Autodesk Inventor part; units mm, degrees
ref_plane "YZ Plane" through (0, 0, 0) normal (1, 0, 0) x (0, 1, 0)
ref_plane "XZ Plane" through (0, 0, 0) normal (0, 1, 0) x (-1, 0, 0)
ref_plane "XY Plane" through (0, 0, 0) normal (0, 0, 1) x (1, 0, 0)
sketch "Sketch1" plane through (0, 0, 0) normal (0, 0, 1) x (1, 0, 0)
  line L0 (0, 0) -> (762, 0)
  line L1 (0, 0) -> (0, -101.6)
  line L2 (0, -101.6) -> (76.2, -101.6)
  line L3 (76.2, -101.6) -> (76.2, -203.2)
  line L4 (76.2, -203.2) -> (0, -203.2)
  line L5 (0, -203.2) -> (0, -266.7)
  line L6 (0, -266.7) -> (228.6, -266.7)
  line L7 (228.6, -266.7) -> (228.6, -355.6)
  line L8 (0, -711.2) -> (762, -711.2)
  line L9 (0, -711.2) -> (0, -609.6)
  line L10 (0, -609.6) -> (76.2, -609.6)
  line L11 (76.2, -609.6) -> (76.2, -508)
  line L12 (76.2, -508) -> (0, -508)
  line L13 (0, -508) -> (0, -444.5)
  line L14 (0, -444.5) -> (228.6, -444.5)
  line L15 (228.6, -444.5) -> (228.6, -355.6)
  line L16 (762, 0) -> (762, -101.6)
  line L17 (762, -101.6) -> (685.8, -101.6)
  line L18 (685.8, -101.6) -> (685.8, -203.2)
  line L19 (685.8, -203.2) -> (762, -203.2)
  line L20 (762, -203.2) -> (762, -266.7)
  line L21 (762, -266.7) -> (533.4, -266.7)
  line L22 (533.4, -266.7) -> (533.4, -355.6)
  line L23 (762, -711.2) -> (762, -609.6)
  line L24 (762, -609.6) -> (685.8, -609.6)
  line L25 (685.8, -609.6) -> (685.8, -508)
  line L26 (685.8, -508) -> (762, -508)
  line L27 (762, -508) -> (762, -444.5)
  line L28 (762, -444.5) -> (533.4, -444.5)
  line L29 (533.4, -444.5) -> (533.4, -355.6)
  dimension "d0" = 762
  dimension "d1" = 101.6
  dimension "d2" = 76.2
  dimension "d3" = 101.6
  dimension "d4" = 63.5
  dimension "d5" = 228.6
  dimension "d7" = 88.9
extrude "Extrusion1" add sketch "Sketch1" along normal blind 9.525
sketch "Sketch2" plane through (0, 0, 9.525) normal (0, 0, 1) x (1, 0, 0)
  line L0 (0, 0) -> (12.7, 0)
  line L1 (0, 0) -> (762, 0)
  line L2 (12.7, 0) -> (12.7, -12.7)
  line L3 (12.7, -12.7) -> (38.1, -12.7)
  line L4 (38.1, -12.7) -> (38.1, -38.1)
  line L5 (38.1, -38.1) -> (12.7, -38.1)
  circle A0 centre (12.7, -12.7) radius 2.54
  circle A1 centre (38.1, -12.7) radius 2.54
  circle A2 centre (38.1, -38.1) radius 2.54
  circle A3 centre (12.7, -38.1) radius 2.54
  line L6 (0, -203.2) -> (76.2, -203.2)
  line L7 (0, -203.2) -> (12.7, -203.2)
  line L8 (12.7, -203.2) -> (12.7, -215.9)
  line L9 (228.6, -266.7) -> (0, -266.7)
  line L10 (0, -266.7) -> (12.7, -266.7)
  line L11 (12.7, -266.7) -> (12.7, -254)
  circle A4 centre (12.7, -254) radius 2.54
  circle A5 centre (12.7, -215.9) radius 2.54
  line L12 (381, 0) -> (381, -711.2)
  line L13 (762, -711.2) -> (0, -711.2)
  line L14 (0, -355.6) -> (762, -355.6)
  line L15 (762, 0) -> (749.3, 0)
  line L16 (762, 0) -> (0, 0)
  line L17 (749.3, 0) -> (749.3, -12.7)
  line L18 (749.3, -12.7) -> (723.9, -12.7)
  line L19 (723.9, -12.7) -> (723.9, -38.1)
  line L20 (723.9, -38.1) -> (749.3, -38.1)
  circle A6 centre (749.3, -12.7) radius 2.54
  circle A7 centre (723.9, -12.7) radius 2.54
  circle A8 centre (723.9, -38.1) radius 2.54
  circle A9 centre (749.3, -38.1) radius 2.54
  line L21 (762, -203.2) -> (685.8, -203.2)
  line L22 (762, -203.2) -> (749.3, -203.2)
  line L23 (749.3, -203.2) -> (749.3, -215.9)
  line L24 (533.4, -266.7) -> (762, -266.7)
  line L25 (762, -266.7) -> (749.3, -266.7)
  line L26 (749.3, -266.7) -> (749.3, -254)
  circle A10 centre (749.3, -254) radius 2.54
  circle A11 centre (749.3, -215.9) radius 2.54
  line L27 (0, -711.2) -> (12.7, -711.2)
  line L28 (0, -711.2) -> (762, -711.2)
  line L29 (12.7, -711.2) -> (12.7, -698.5)
  line L30 (12.7, -698.5) -> (38.1, -698.5)
  line L31 (38.1, -698.5) -> (38.1, -673.1)
  line L32 (38.1, -673.1) -> (12.7, -673.1)
  circle A12 centre (12.7, -698.5) radius 2.54
  circle A13 centre (38.1, -698.5) radius 2.54
  circle A14 centre (38.1, -673.1) radius 2.54
  circle A15 centre (12.7, -673.1) radius 2.54
  line L33 (0, -508) -> (76.2, -508)
  line L34 (0, -508) -> (12.7, -508)
  line L35 (12.7, -508) -> (12.7, -495.3)
  line L36 (228.6, -444.5) -> (0, -444.5)
  line L37 (0, -444.5) -> (12.7, -444.5)
  line L38 (12.7, -444.5) -> (12.7, -457.2)
  circle A16 centre (12.7, -457.2) radius 2.54
  circle A17 centre (12.7, -495.3) radius 2.54
  line L39 (381, -711.2) -> (381, 0)
  line L40 (762, -711.2) -> (749.3, -711.2)
  line L41 (762, -711.2) -> (0, -711.2)
  line L42 (749.3, -711.2) -> (749.3, -698.5)
  line L43 (749.3, -698.5) -> (723.9, -698.5)
  line L44 (723.9, -698.5) -> (723.9, -673.1)
  line L45 (723.9, -673.1) -> (749.3, -673.1)
  circle A18 centre (749.3, -698.5) radius 2.54
  line L46 (533.4, -444.5) -> (762, -444.5)
  line L47 (749.3, -444.5) -> (749.3, -457.2)
  line L48 (762, -444.5) -> (749.3, -444.5)
  circle A19 centre (749.3, -457.2) radius 2.54
  circle A20 centre (749.3, -495.3) radius 2.54
  line L49 (749.3, -508) -> (749.3, -495.3)
  line L50 (762, -508) -> (685.8, -508)
  line L51 (762, -508) -> (749.3, -508)
  circle A21 centre (723.9, -673.1) radius 2.54
  circle A22 centre (723.9, -698.5) radius 2.54
  circle A23 centre (749.3, -673.1) radius 2.54
  dimension "d10" = 12.7
  dimension "d11" = 12.7
  dimension "d12" = 25.4
  dimension "d13" = 25.4
  dimension "d14" = 25.4
  dimension "d16" = 5.08
  dimension "d17" = 12.7
  dimension "d18" = 12.7
  dimension "d19" = 12.7
extrude "Extrusion2" cut sketch "Sketch2" against normal blind 9.525
sketch "Sketch4" plane through (0, 0, 9.525) normal (0, 0, 1) x (1, 0, 0)
  circle A0 centre (38.1, -12.7) radius 2.54
  line L0 (38.1, -12.7) -> (63.5, -12.7) construction
  line L1 (63.5, -12.7) -> (88.9, -12.7) construction
  circle A1 centre (63.5, -12.7) radius 2.54
  circle A2 centre (88.9, -12.7) radius 2.54
  line L2 (762, 0) -> (0, 0)
  line L3 (0, -711.2) -> (762, -711.2)
  line L4 (0, -355.6) -> (799.6249, -355.6)
  line L5 (723.9, -12.7) -> (698.5, -12.7) construction
  line L6 (698.5, -12.7) -> (673.1, -12.7) construction
  circle A3 centre (698.5, -12.7) radius 2.54
  circle A4 centre (673.1, -12.7) radius 2.54
  line L7 (381, 0) -> (381, -12.7)
  circle A5 centre (381, -12.7) radius 2.54
  line L8 (38.1, -698.5) -> (63.5, -698.5) construction
  line L9 (63.5, -698.5) -> (88.9, -698.5) construction
  circle A6 centre (63.5, -698.5) radius 2.54
  circle A7 centre (88.9, -698.5) radius 2.54
  line L10 (723.9, -698.5) -> (698.5, -698.5) construction
  line L11 (698.5, -698.5) -> (673.1, -698.5) construction
  circle A8 centre (698.5, -698.5) radius 2.54
  circle A9 centre (673.1, -698.5) radius 2.54
  circle A10 centre (381, -698.5) radius 2.54
  dimension "d29" = 25.4
  dimension "d30" = 25.4
  dimension "d32" = 12.7
extrude "Extrusion4" cut sketch "Sketch4" against normal blind 25.4 contours A1 | A2 | A3 | A4 | A5 | A6 | A7 | A8 | A9 | A10
properties part number "Belly Pan V2"
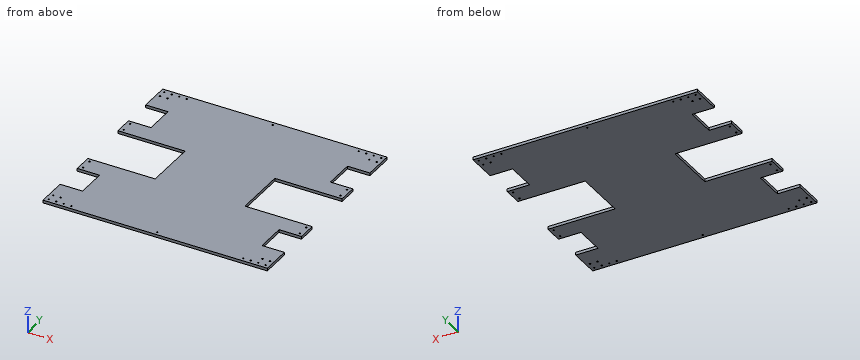
Build history of the part. All positions in model axes, mm. Give positions to 0.01 mm unless a question says otherwise; leave off trailing zeros. Order: outer loops, then holes, each group sorted by start corner. A loop starts at its lowest first (then second) coordinate and runs counter-clockwise, first axis right, second up. Notation, with made-up numbers: M 56,-1 L 92,-1 A24 cw 92,36 Z; hole C -15,53.5 d1. An arc over 180 degrees is marked long. Use one line per item in the form item = value.
1) Saw through at A-A (x = 602). Give the cut face in (y, z) (3 decimals).
Calculated:
outline = M -711.2,0 L -444.5,0 L -444.5,9.525 L -711.2,9.525 Z; M -266.7,0 L 0,0 L 0,9.525 L -266.7,9.525 Z
2) Probe probe 1 along X at (y, z) = (-254, 3); probe 2 along Y at (x, z) = (48, 5); probe 3 along Y at (x, z) = (698.5, 2). List the from-to ranges inside material, lowest first.
Calculated:
probe_1 = 0 to 10.16, 15.24 to 746.76, 751.84 to 762
probe_2 = -711.2 to -609.6, -508 to -444.5, -266.7 to -203.2, -101.6 to 0
probe_3 = -711.2 to -701.04, -695.96 to -609.6, -508 to -444.5, -266.7 to -203.2, -101.6 to -15.24, -10.16 to 0
3) Saw through at C-C (y = -111). Give the cut face in (x, z) (3 decimals).
Calculated:
outline = M 76.2,0 L 685.8,0 L 685.8,9.525 L 76.2,9.525 Z
4) Saw through at B-B (z = 7). State how many separate pieces and enclosed holes the cut face has, plus the area to 3 significant figures.
Calculated:
separate_pieces = 1
enclosed_holes = 34
area = 429,000 mm2
5) Drop flat-ended pins along their axis: pin 1 (1.5 mm diameter, centred on y = -313.5, z = 5, fed in from -X); pin 2 (4 mm diameter, centred on x = 673.1, y = -12.7, fed in from +Z); pin 3 (5 mm diameter, centred on y = -108, z = 5.5, fed in from +X). Give the stop position or say it passes through.
Calculated:
pin_1 = 228.6
pin_2 = through
pin_3 = 685.8
